```python
from build123d import *

# Parameters (mm, degrees)
EXTRUDE_2_DEPTH     = 5
SKETCH_4_R          = 4
CUT_EXTRUDE_1_DEPTH = 5
SKETCH_6_R          = 12.5
EXTRUDE_3_DEPTH     = 5
SKETCH_8_R          = 7.5
CUT_EXTRUDE_2_DEPTH = 5


with BuildPart() as part:
    # 草图3 → 凸台-拉伸2 (new body)
    with BuildSketch(Plane(origin=(0, 0, 0), x_dir=(1, 0, 0), z_dir=(0, 1, 0))):
        with BuildLine():
            Line((0, -12.5), (-30, -12.5))
            Line((-30, -12.5), (-30, -6.5))
            Line((-30, -6.5), (-18, -6.5))
            Line((-18, -6.5), (-18, 6.5))
            Line((-18, 6.5), (-30, 6.5))
            Line((-30, 6.5), (-30, 12.5))
            Line((-30, 12.5), (0, 12.5))
            ThreePointArc((0, 12.5), (4.453089161, 11.679897128), (8.321859729, 9.327199507))
            Line((8.321859729, 9.327199507), (20.301898362, 16.813158484))
            ThreePointArc((20.301898362, 16.813158484), (31.377779558, 19.607012777), (24.011333212, 10.876821811))
            Line((24.011333212, 10.876821811), (12.031294579, 3.390862834))
            ThreePointArc((12.031294579, 3.390862834), (9.965836278, -7.545336791), (0, -12.5))
        make_face()
    extrude(amount=EXTRUDE_2_DEPTH)

    # 草图4 → 切除-拉伸1 (cut)
    with BuildSketch(Plane(origin=(0, 0, 0), x_dir=(1, 0, 0), z_dir=(0, 1, 0))):
        with Locations(Location((26.289490981, 16.427497191, 0), (0, 0, 270))):
            Circle(SKETCH_4_R)
    extrude(amount=CUT_EXTRUDE_1_DEPTH, mode=Mode.SUBTRACT)

    # 草图6 → 凸台-拉伸3 (add)
    with BuildSketch(Plane(origin=(0, 5, 0), x_dir=(1, 0, 0), z_dir=(0, 1, 0))):
        with Locations(Location((0, 0, 0), (0, 0, 270))):
            Circle(SKETCH_6_R)
    extrude(amount=EXTRUDE_3_DEPTH)

    # 草图8 → 切除-拉伸2 (cut, symmetric)
    with BuildSketch(Plane(origin=(0, 5, 0), x_dir=(1, 0, 0), z_dir=(0, 1, 0))):
        with Locations(Location((0, 0, 0), (0, 0, 270))):
            Circle(SKETCH_8_R)
    extrude(amount=CUT_EXTRUDE_2_DEPTH, both=True, mode=Mode.SUBTRACT)


solid = part.part
```
Here's how the part is built. I have some questions about the finished solid (model axes, mm). A direction names the side the tool comes from. Round coordinates to 2 decimals unless told otherwise and drop trailing zeros. Order: outer loops, then holes, each group sorted by start corner. A loop starts at its lowest first (then second) coordinate and runs counter-clockwise, first axis right, second up. Notation, with made-up numbers: M -33,-7 L -8,-7 A34 cw -8,26 Z; hole C 37,51 d3. An arc over 180 degrees is marked long. One line per question, with ' | ' between items.
1) I want a section at B-B, the plane y = 4.25. Write out the boundary of the cut face in (x, z), then the cut area to 3 significant figures.
Working result:
outline: M -30,-12.5 L 0,-12.5 A12.5 ccw 8.32,-9.33 L 20.3,-16.81 A6 ccw long 24.01,-10.88 L 12.03,-3.39 A12.5 ccw 0,12.5 L -30,12.5 L -30,6.5 L -18,6.5 L -18,-6.5 L -30,-6.5 Z; hole C 0,0 d15; hole C 26.29,-16.43 d8 | area: 817 mm²
2) I want a section at C-C, the plane z = 4. Write out the boundary of the cut face in (x, y).
Working result:
outline: M -18,0 L -6.34,0 L -6.34,10 L -11.84,10 L -11.84,5 L -18,5 Z; M 6.34,0 L 11.84,0 L 11.84,10 L 6.34,10 Z
3) I want a section at A-A, the plane z = 0. Write out the boundary of the cut face in (x, y).
Working result:
outline: M -18,0 L -7.5,0 L -7.5,10 L -12.5,10 L -12.5,5 L -18,5 Z; M 7.5,0 L 12.5,0 L 12.5,10 L 7.5,10 Z
4) If we mould it in two halves opening along X, with no side actions, what happens to faces 1 (the face through (0.33, 5.07, -7.493)), 2 (the face through (-30, 2, 10)), 3 (the face through (-24, 2, 6.5)), 4 (the face through (23.856, 2.465, -19.602))? For each: +X half, -X half, draft (parallel to the pull), parting line (faces both ways), or undercut.
Working result:
face 1: undercut | face 2: -X half | face 3: draft | face 4: undercut
5) For faces 5 (the face through (14.2, 2.5, -13)), 6 (the face through (-18, 2, 0)), 7 (the face through (-15, 5, 0)), which set-ups out of +Z, -Z, +X, -X, +Y, -Y let a thin tool reach every point of the face, with its end or its side?
Working result:
face 5: -Z, +Y, -Y | face 6: -X, +Y, -Y | face 7: -X, +Y
6) For pin 1 Ø1 at (x, y) = (12.5, 3.5) entering from -Z; pin 2 Ø4 at (x, y) = (-17, 2) entering from -Z; pin 3 Ø12 at (x, z) = (-15, -17.5) entering from +Y, each with a flat end and sliding along its axis, tell me the tip position at first contact or that it passes through.
Working result:
pin 1: z = -12.25 | pin 2: z = -12.5 | pin 3: y = 5
7) I need wall thicknesses on line 1 along Y through (x, z) = (-6.5, -12); line 2 along X through (y, z) = (4, -17); line 3 along Z through (x, y) = (-10, 6). Which ranges of each line are inside material? Lowest first, please.
Working result:
line 1: 0 to 5 | line 2: 20.32 to 22.33, 30.25 to 32.26 | line 3: -7.5 to 7.5
